Can you work these out from the model? Positions are in its coordinate system, mm. Face numbers are marked on the shaded views. A direction names the side the tool comes from. Coordinates: 2 decimals unless noted, no trailing zeros. Write each loop counter-clockwise with the first axis right and the second up, starting at its lowest first coordinate (ties: lowest second). Pieces come first, ordered by that corner, then holes. Notation, with made-up numbers: (85, -39) -> (118, -39) arc R31 cw to (118, -7) -> close; hole circle Ø2 at (61.25, 65.25). An arc over 180 degrees is marked (long way). Use one line per item in the form item = value.
```python
from build123d import *

# Parameters (mm, degrees)
ESBO_O1_W                = 93
ESBO_O1_H                = 49
RESSALTO_EXTRUS_O1_DEPTH = 1.26
ESBO_O2_W                = 93
ESBO_O2_H                = 1.26
RESSALTO_EXTRUS_O2_DEPTH = 35.24
ESBO_O3_W                = 1.26
ESBO_O3_H                = 49
RESSALTO_EXTRUS_O4_DEPTH = 35.24
RESSALTO_EXTRUS_O5_START = 35
RESSALTO_EXTRUS_O5_DEPTH = 57
FILETE1_R                = 1
FILETE2_R                = 1
ESBO_O6_W                = 1.26
ESBO_O6_H                = 49
RESSALTO_EXTRUS_O6_DEPTH = 33.98
ESBO_O7_W                = 11
ESBO_O7_H                = 2
CORTE_EXTRUS_O1_DEPTH    = 1.26
ESBO_O8_W                = 13
ESBO_O8_H                = 2
CORTE_EXTRUS_O2_DEPTH    = 1.26
RESSALTO_EXTRUS_O7_DEPTH = 2
RESSALTO_EXTRUS_O8_DEPTH = 2


with BuildPart() as part:
    # Esboço1 → Ressalto-extrusão1 (new body)
    with BuildSketch(Plane(origin=(0, 0, 0), x_dir=(1, 0, 0), z_dir=(0, 1, 0))):
        with Locations((46.5, -24.5)):
            Rectangle(ESBO_O1_W, ESBO_O1_H)
    extrude(amount=RESSALTO_EXTRUS_O1_DEPTH)

    # Esboço2 → Ressalto-extrusão2 (add)
    with BuildSketch(Plane(origin=(0, 0, 0), x_dir=(1, 0, 0), z_dir=(0, 1, 0))):
        with Locations((46.5, -0.63)):
            Rectangle(ESBO_O2_W, ESBO_O2_H)
        with Locations((46.5, -48.37)):
            Rectangle(ESBO_O2_W, ESBO_O2_H)
    extrude(amount=RESSALTO_EXTRUS_O2_DEPTH)

    # Esboço3 → Ressalto-extrusão4 (add)
    with BuildSketch(Plane(origin=(0, 0, 0), x_dir=(1, 0, 0), z_dir=(0, 1, 0))):
        with Locations((92.37, -24.5)):
            Rectangle(ESBO_O3_W, ESBO_O3_H)
    extrude(amount=RESSALTO_EXTRUS_O4_DEPTH)

    # Esboço5 → Ressalto-extrusão5 (add)
    with BuildSketch(Plane(origin=(0, 0, 0), x_dir=(0, 0, -1), z_dir=(1, 0, 0)).offset(RESSALTO_EXTRUS_O5_START)):
        Polygon((0, 35.24), (-3.26, 35.24), (0, 31.98), align=None)
        Polygon((-49, 35.24), (-45.74, 35.24), (-49, 31.98), align=None)
    extrude(amount=RESSALTO_EXTRUS_O5_DEPTH)

    # Filete1
    filete1_edges = [part.edges().sort_by_distance(p)[0] for p in [
        (35, 34.24, 46.74),
    ]]
    fillet(filete1_edges, radius=FILETE1_R)

    # Filete2
    filete2_edges = [part.edges().sort_by_distance(p)[0] for p in [
        (35, 34.24, 2.26),
    ]]
    fillet(filete2_edges, radius=FILETE2_R)

    # Esboço6 → Ressalto-extrusão6 (add)
    with BuildSketch(Plane(origin=(0, 0, 0), x_dir=(1, 0, 0), z_dir=(0, 1, 0))):
        with Locations((0.63, -24.5)):
            Rectangle(ESBO_O6_W, ESBO_O6_H)
    extrude(amount=RESSALTO_EXTRUS_O6_DEPTH)

    # Esboço7 → Corte-extrusão1 (cut)
    with BuildSketch(Plane.ZY):
        with Locations((24.5, 2.26)):
            Rectangle(ESBO_O7_W, ESBO_O7_H)
    extrude(amount=-CORTE_EXTRUS_O1_DEPTH, mode=Mode.SUBTRACT)

    # Esboço8 → Corte-extrusão2 (cut)
    with BuildSketch(Plane(origin=(93, 0, 0), x_dir=(0, 0, -1), z_dir=(1, 0, 0))):
        with Locations((-24.5, 2.26)):
            Rectangle(ESBO_O8_W, ESBO_O8_H)
    extrude(amount=-CORTE_EXTRUS_O2_DEPTH, mode=Mode.SUBTRACT)

    # Esboço10 → Ressalto-extrusão7 (add)
    with BuildSketch(Plane(origin=(0, 1.26, 0), x_dir=(1, 0, 0), z_dir=(0, 1, 0))):
        Polygon((4, -15.74), (4, -17), (8, -17), (8, -19), (9.26, -19), (9.26, -15.74), align=None)
        Polygon((4, -32), (4, -33.26), (9.26, -33.26), (9.26, -30), (8, -30), (8, -32), align=None)
    extrude(amount=RESSALTO_EXTRUS_O7_DEPTH)

    # Esboço11 → Ressalto-extrusão8 (add)
    with BuildSketch(Plane(origin=(0, 1.26, 0), x_dir=(1, 0, 0), z_dir=(0, 1, 0))):
        Polygon((87.74, -14.24), (83.74, -14.24), (83.74, -17.5), (85, -17.5), (85, -15.5), (87.74, -15.5), align=None)
        Polygon((87.74, -33.5), (87.74, -34.76), (83.74, -34.76), (83.74, -31.5), (85, -31.5), (85, -33.5), align=None)
    extrude(amount=RESSALTO_EXTRUS_O8_DEPTH)


solid = part.part
```
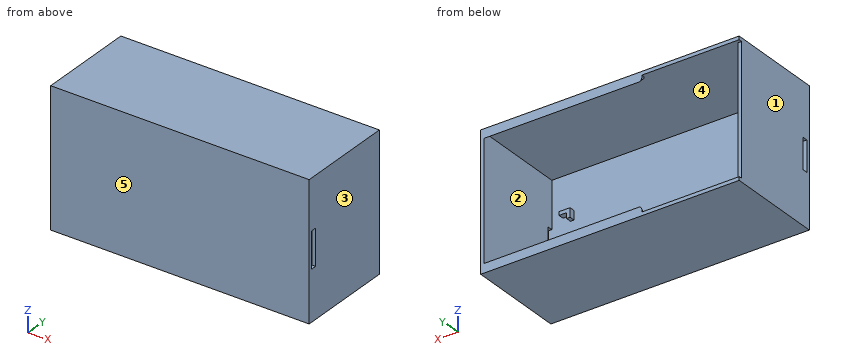
Q1. Suppose I cut it at A-A (z = 20.5). Write out the boundary of the cut face in (x, y), then the cut area to 3 significant figures.
Return value:
outline = (0, 0) -> (93, 0) -> (93, 1.26) -> (0, 1.26) -> close; (0, 3.26) -> (1.26, 3.26) -> (1.26, 33.98) -> (0, 33.98) -> close; (91.74, 3.26) -> (93, 3.26) -> (93, 35.24) -> (91.74, 35.24) -> close
area = 196 mm2
Q2. For the marked faces 4 and 5, which set-ups out of +Z, -Z, +X, -X, +Y, -Y let a thin tool reach every point of the face, with its end or its side?
Return value:
face_4 = none
face_5 = +Z, -Z, +X, -X, -Y
Q3. Suppose I cut it at B-B (y = 5.5). Write out the boundary of the cut face in (x, z).
Return value:
outline = (0, 0) -> (93, 0) -> (93, 49) -> (0, 49) -> close; hole (1.26, 1.26) -> (91.74, 1.26) -> (91.74, 47.74) -> (1.26, 47.74) -> close
Q4. Thinking about a two-plate mould opening in X: for the marked faces 1, 2 and 3, which applies, released by +X, released by -X, zero draft, split by the parting line, or undercut?
Return value:
face_1 = released by -X
face_2 = undercut
face_3 = released by +X
Q5. Suppose I cut it at C-C (x = 63). Write out the boundary of the cut face in (y, z), then the cut area to 3 significant figures.
Return value:
outline = (0, 0) -> (35.24, 0) -> (35.24, 3.26) -> (33.24, 1.26) -> (1.26, 1.26) -> (1.26, 47.74) -> (33.24, 47.74) -> (35.24, 45.74) -> (35.24, 49) -> (0, 49) -> close
area = 151 mm2
Q6. Suppose I cut it at D-D (z = 40). Write out the boundary of the cut face in (x, y).
Return value:
outline = (0, 0) -> (93, 0) -> (93, 35.24) -> (91.74, 35.24) -> (91.74, 1.26) -> (1.26, 1.26) -> (1.26, 33.98) -> (0, 33.98) -> close
Q7. If I drill on line 1 (Z direction, x = 12.5, y = 10.5); line 2 (X direction, y = 22.5, z = 47); line 3 (Y direction, x = 58, z = 17), over which ranges is the centre line in solid material (lowest first)? Write a range as from..to.
Return value:
line_1 = 0..1.26, 47.74..49
line_2 = 0..1.26, 91.74..93
line_3 = 0..1.26
Q8. Will these pins go through, and if not, where does the flat tip stop? pin 1 (1.6 mm diameter, centred on y = 2.5, z = 33.5, fed in from -X); pin 2 (3.5 mm diameter, centred on x = 7, z = 32.5, fed in from +Y); pin 3 (2 mm diameter, centred on x = 66.5, z = 9, fed in from +Y).
Return value:
pin_1 = 0
pin_2 = 3.26
pin_3 = 1.26
